Read the model definition and answer for the solid it produces. Units are mm, in the model's axes. A direction names the side the tool comes from. Give positions to 0.01 mm unless a question says otherwise; leave off trailing zeros. Loops run counter-clockwise (first coordinate to the right, second up) from the corner with the lowest first, then second, coordinate; pieces in that order, holes last. Notation, with made-up numbers: (63.5, -26.5) - (103.5, -26.5) arc R33 cw to (103.5, 1.5) - close; hole circle Ø9 at (69, 42.25). An arc over 180 degrees is marked (long way). Put each result on its own line as item: value. Start each with the question number.
1. A cutting plane is placed at B-B, the plane z = 2.4. Determine the outline of the cut face in (x, y) (3 decimals), plus the area to 3 significant figures.
2. For a pull along Y with two mould halves and no side action, classify faces 1 (the flat face through (424.744, -13, 2)), 2 (the flat face through (434, 0, 2)), 3 (the cylindrical face through (454.665, -25.203, 1.503)) as released by +Y, released by -Y, zero draft, split by the parting line, or undercut.
3. Consider L1, parallel to Y at x = 427, z = 2.6 (3 decimals); L2, parallel to X at y = -25.5, z = 1.05; L3, parallel to Y at x = 453, z = 0.85. Determine where each line is inside the solid, lowest interval first. Write a range as from..to.
4. Given pin 1 Ø1.5 at (y, z) = (-33.5, 1.5) entering from +X (3 decimals); pin 2 Ø1.5 at (y, z) = (-1, 1) entering from -X; pin 3 Ø0.9 at (x, z) = (426.5, 1.5) entering from +Y (3 decimals), each flat-ended and moving along its own axis, determine where each tip first touches the part or whether it passes through.
5. A cutting plane is placed at A-A, the plane x = 452.5. Determine the outline of the cut face in (y, z), plus the area to 3 significant figures.
6. A cutting plane is placed at C-C, the plane y = -23.5. Determine the outline of the cut face in (x, z), plus the area to 3 significant figures.
7. A cutting plane is placed at D-D, the plane y = -31.5. Determine the outline of the cut face in (x, z), plus the area to 3 significant figures.
8. For faces 4 (the flat face through (445, -19, 3.048)), 5 (the flat face through (426, -22.225, 2)), 6 (the flat face through (427.919, -2, 2)), determine the directions among +Z, -Z, +X, -X, +Y, -Y from which every point of the face is accessible in a straight line to the end or side of a thin tool.
```python
from build123d import *

# Parameters (mm, degrees)
SKETCH1_R           = 3.3
BOSS_EXTRUDE1_DEPTH = 3.048


with BuildPart() as part:
    # Sketch1 → Boss-Extrude1 (new body)
    with BuildSketch(Plane.XY):
        with BuildLine():
            Line((427.919423357, 0), (440.619423357, 0))
            Line((440.619423357, 0), (461.432219063, -17.609164677))
            ThreePointArc((461.432219063, -17.609164677), (462.308947418, -31.354922495), (450.144423357, -37.815484776))
            Line((450.144423357, -37.815484776), (427.919423357, -25.4))
            Line((427.919423357, -25.4), (427.919423357, -22.225))
            Line((427.919423357, -22.225), (424.744423357, -22.225))
            Line((424.744423357, -22.225), (424.744423357, -3.175))
            Line((424.744423357, -3.175), (427.919423357, -3.175))
            Line((427.919423357, -3.175), (427.919423357, 0))
        make_face()
        with Locations(Location((451.368205009, -25.058241389, 0), (0, 0, 180))):
            Circle(SKETCH1_R, mode=Mode.SUBTRACT)
    extrude(amount=BOSS_EXTRUDE1_DEPTH)


solid = part.part
```
Return value:
1. outline: (424.744, -22.225) - (427.919, -22.225) - (427.919, -25.4) - (450.144, -37.815) arc R12.7 ccw to (461.432, -17.609) - (440.619, 0) - (427.919, 0) - (427.919, -3.175) - (424.744, -3.175) - close; hole circle Ø6.6 at (451.368, -25.058)
1. area: 983 mm2
2. face 1: zero draft
2. face 2: released by +Y
2. face 3: undercut
3. L1: y = -22.225..-3.175
3. L2: x = 428.1..448.1, 454.64..463.92
3. L3: y = -37.74..-27.93, -22.19..-10.47
4. pin 1: stops at x = 461.405
4. pin 2: stops at x = 427.92
4. pin 3: stops at y = -3.175
5. outline: (-37.8, 0) - (-28.16, 0) - (-28.16, 3.05) - (-37.8, 3.05) - close; (-21.96, 0) - (-10.05, 0) - (-10.05, 3.05) - (-21.96, 3.05) - close
5. area: 65.7 mm2
6. outline: (427.92, 0) - (448.46, 0) - (448.46, 3.05) - (427.92, 3.05) - close; (454.28, 0) - (463.81, 0) - (463.81, 3.05) - (454.28, 3.05) - close
6. area: 91.7 mm2
7. outline: (438.84, 0) - (462.23, 0) - (462.23, 3.05) - (438.84, 3.05) - close
7. area: 71.3 mm2
8. face 4: +Z, +X, -X, +Y, -Y
8. face 5: +Z, -Z, -X, -Y
8. face 6: +Z, -Z, -X, +Y
